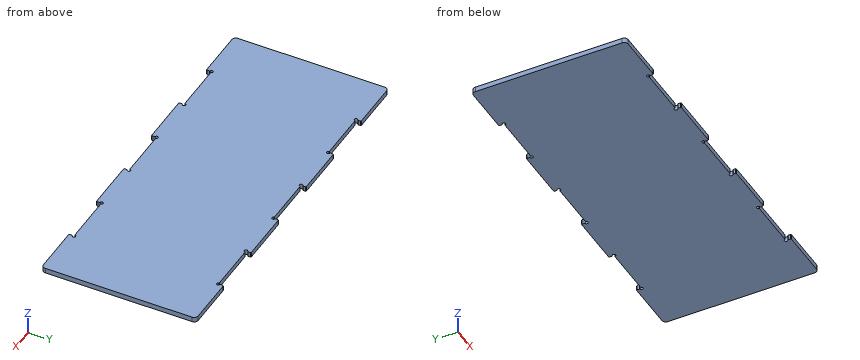
```python
from build123d import *

# Parameters (mm, degrees)
SKETCH1_W               = 455
SKETCH1_H               = 180
BOSS_EXTRUDE1_DEPTH     = 3.175
SKETCH2_W               = 65
SKETCH2_H               = 6.35
BOSS_EXTRUDE2_DEPTH     = 6.35
LPATTERN1_COUNT         = 4
LPATTERN1_PITCH         = 130
MIRROR1_COPY_1_SKETCH_W = 65
MIRROR1_COPY_1_SKETCH_H = 6.35
MIRROR1_COPY_1_DEPTH    = 6.35
MIRROR1_COPY_2_SKETCH_W = 65
MIRROR1_COPY_2_SKETCH_H = 6.35
MIRROR1_COPY_2_DEPTH    = 6.35
MIRROR1_COPY_3_SKETCH_W = 65
MIRROR1_COPY_3_SKETCH_H = 6.35
MIRROR1_COPY_3_DEPTH    = 6.35
SKETCH3_R               = 2
CUT_EXTRUDE1_DEPTH      = 7.35
FILLET2_R               = 1
CUT_EXTRUDE2_DEPTH      = 7.35
LPATTERN2_COUNT         = 3
LPATTERN2_PITCH         = 130
MIRROR2_COPY_1_DEPTH    = 7.35
MIRROR2_COPY_2_DEPTH    = 7.35
FILLET4_R               = 5


with BuildPart() as part:
    # Sketch1 → Boss-Extrude1 (new body, symmetric)
    with BuildSketch(Plane.XY):
        with Locations((227.5, 90)):
            Rectangle(SKETCH1_W, SKETCH1_H)
    extrude(amount=BOSS_EXTRUDE1_DEPTH, both=True)

    # Sketch2 → Boss-Extrude2 (add)
    with BuildSketch(Plane.XY.offset(3.175)):
        with Locations((422.5, -3.175)):
            Rectangle(SKETCH2_W, SKETCH2_H)
    boss_extrude2 = extrude(amount=-BOSS_EXTRUDE2_DEPTH)

    # LPattern1: Boss-Extrude2 ×4
    with Locations(*[(-i * LPATTERN1_PITCH, 0, 0) for i in range(1, LPATTERN1_COUNT)]):
        add(boss_extrude2)

    # Mirror1: Boss-Extrude2 across plane
    add(boss_extrude2.mirror(Plane(origin=(0, 90, 0), x_dir=(0, 0, 1), z_dir=(0, -1, 0))))

    # Mirror1 copy 1 sketch → Mirror1 copy 1 (add)
    with BuildSketch(Plane(origin=(-130, 180, 3.175), x_dir=(1, 0, 0), z_dir=(0, 0, 1))):
        with Locations((422.5, 3.175)):
            Rectangle(MIRROR1_COPY_1_SKETCH_W, MIRROR1_COPY_1_SKETCH_H)
    extrude(amount=-MIRROR1_COPY_1_DEPTH)

    # Mirror1 copy 2 sketch → Mirror1 copy 2 (add)
    with BuildSketch(Plane(origin=(-260, 180, 3.175), x_dir=(1, 0, 0), z_dir=(0, 0, 1))):
        with Locations((422.5, 3.175)):
            Rectangle(MIRROR1_COPY_2_SKETCH_W, MIRROR1_COPY_2_SKETCH_H)
    extrude(amount=-MIRROR1_COPY_2_DEPTH)

    # Mirror1 copy 3 sketch → Mirror1 copy 3 (add)
    with BuildSketch(Plane(origin=(-390, 180, 3.175), x_dir=(1, 0, 0), z_dir=(0, 0, 1))):
        with Locations((422.5, 3.175)):
            Rectangle(MIRROR1_COPY_3_SKETCH_W, MIRROR1_COPY_3_SKETCH_H)
    extrude(amount=-MIRROR1_COPY_3_DEPTH)

    # Sketch3 → Cut-Extrude1 (cut, through all)
    with BuildSketch(Plane.XY.offset(3.175)):
        with Locations((325, 0)):
            Circle(SKETCH3_R)
        with Locations((390, 0)):
            Circle(SKETCH3_R)
    extrude(amount=-CUT_EXTRUDE1_DEPTH, mode=Mode.SUBTRACT)

    # Fillet2
    fillet2_edges = [part.edges().sort_by_distance(p)[0] for p in [
        (390, -6.35, 0),
        (325, -6.35, 0),
    ]]
    fillet(fillet2_edges, radius=FILLET2_R)

    # Sketch4 → Cut-Extrude2 (cut, through all)
    with BuildSketch(Plane.XY.offset(3.175)):
        with BuildLine():
            Line((390, -2.828427125), (390, -5.35))
            ThreePointArc((390, -5.35), (390.292893219, -6.057106781), (391, -6.35))
            Line((391, -6.35), (324, -6.35))
            ThreePointArc((324, -6.35), (324.707106781, -6.057106781), (325, -5.35))
            Line((325, -5.35), (325, -2.828427125))
            ThreePointArc((325, -2.828427125), (324.816496581, -2.251076856), (324.333333333, -1.885618083))
            ThreePointArc((324.333333333, -1.885618083), (323.585786438, 1.414213562), (326.885618083, 0.666666667))
            ThreePointArc((326.885618083, 0.666666667), (327.251076856, 0.183503419), (327.828427125, 0))
            Line((327.828427125, 0), (387.171572875, 0))
            ThreePointArc((387.171572875, 0), (387.748923144, 0.183503419), (388.114381917, 0.666666667))
            ThreePointArc((388.114381917, 0.666666667), (391.414213562, 1.414213562), (390.666666667, -1.885618083))
            ThreePointArc((390.666666667, -1.885618083), (390.183503419, -2.251076856), (390, -2.828427125))
        make_face()
    cut_extrude2 = extrude(amount=-CUT_EXTRUDE2_DEPTH, mode=Mode.SUBTRACT)

    # LPattern2: Cut-Extrude2 ×3
    with Locations(*[(-i * LPATTERN2_PITCH, 0, 0) for i in range(1, LPATTERN2_COUNT)]):
        add(cut_extrude2, mode=Mode.SUBTRACT)

    # Mirror2: Cut-Extrude2 across plane
    add(cut_extrude2.mirror(Plane(origin=(0, 90, 0), x_dir=(0, 0, 1), z_dir=(0, -1, 0))), mode=Mode.SUBTRACT)

    # Mirror2 copy 1 sketch → Mirror2 copy 1 (cut, through all)
    with BuildSketch(Plane(origin=(-130, 180, 3.175), x_dir=(1, 0, 0), z_dir=(0, 0, 1))):
        with BuildLine():
            Line((390, 2.828427125), (390, 5.35))
            ThreePointArc((390, 5.35), (390.292893219, 6.057106781), (391, 6.35))
            Line((391, 6.35), (324, 6.35))
            ThreePointArc((324, 6.35), (324.707106781, 6.057106781), (325, 5.35))
            Line((325, 5.35), (325, 2.828427125))
            ThreePointArc((325, 2.828427125), (324.816496581, 2.251076856), (324.333333333, 1.885618083))
            ThreePointArc((324.333333333, 1.885618083), (323.585786438, -1.414213562), (326.885618083, -0.666666667))
            ThreePointArc((326.885618083, -0.666666667), (327.251076856, -0.183503419), (327.828427125, 0))
            Line((327.828427125, 0), (387.171572875, 0))
            ThreePointArc((387.171572875, 0), (387.748923144, -0.183503419), (388.114381917, -0.666666667))
            ThreePointArc((388.114381917, -0.666666667), (391.414213562, -1.414213562), (390.666666667, 1.885618083))
            ThreePointArc((390.666666667, 1.885618083), (390.183503419, 2.251076856), (390, 2.828427125))
        make_face()
    extrude(amount=-MIRROR2_COPY_1_DEPTH, mode=Mode.SUBTRACT)

    # Mirror2 copy 2 sketch → Mirror2 copy 2 (cut, through all)
    with BuildSketch(Plane(origin=(-260, 180, 3.175), x_dir=(1, 0, 0), z_dir=(0, 0, 1))):
        with BuildLine():
            Line((390, 2.828427125), (390, 5.35))
            ThreePointArc((390, 5.35), (390.292893219, 6.057106781), (391, 6.35))
            Line((391, 6.35), (324, 6.35))
            ThreePointArc((324, 6.35), (324.707106781, 6.057106781), (325, 5.35))
            Line((325, 5.35), (325, 2.828427125))
            ThreePointArc((325, 2.828427125), (324.816496581, 2.251076856), (324.333333333, 1.885618083))
            ThreePointArc((324.333333333, 1.885618083), (323.585786438, -1.414213562), (326.885618083, -0.666666667))
            ThreePointArc((326.885618083, -0.666666667), (327.251076856, -0.183503419), (327.828427125, 0))
            Line((327.828427125, 0), (387.171572875, 0))
            ThreePointArc((387.171572875, 0), (387.748923144, -0.183503419), (388.114381917, -0.666666667))
            ThreePointArc((388.114381917, -0.666666667), (391.414213562, -1.414213562), (390.666666667, 1.885618083))
            ThreePointArc((390.666666667, 1.885618083), (390.183503419, 2.251076856), (390, 2.828427125))
        make_face()
    extrude(amount=-MIRROR2_COPY_2_DEPTH, mode=Mode.SUBTRACT)

    # Fillet4
    fillet4_edges = [part.edges().sort_by_distance(p)[0] for p in [
        (455, -6.35, 0),
        (0, -6.35, 0),
        (455, 186.35, 0),
        (0, 186.35, 0),
    ]]
    fillet(fillet4_edges, radius=FILLET4_R)


solid = part.part
```
Build history of the part. All positions in model axes, mm. Round coordinates to 2 decimals unless told otherwise and drop trailing zeros. Write each loop counter-clockwise with the first axis right and the second up, starting at its lowest first coordinate (ties: lowest second). Pieces come first, ordered by that corner, then holes.
1) Drill centre line: probe 1 along Y at (x, z) = (90, -1.75). Where is it in solid material? Low to high.
2) Pin check, flat tips, straight feed: pin 1 (0.8 mm diameter, centred on y = 184.5, z = 0.5, fed in from -X); pin 2 (3.5 mm diameter, centred on x = 195, y = 0, fed in from -Z); pin 3 (1.3 mm diameter, centred on y = 184, z = 0.5, fed in from -X); pin 4 (0.8 mm diameter, centred on y = 183.5, z = -0.5, fed in from +X). Stop position of each tip, or through.
3) Band-saw the part on A-A, the plane x = 73. List the corners of the cut face in (y, z) (3 decimals).
Ans:
1. probe 1: y = 0 to 180
2. pin 1: stops at x = 0.82
2. pin 2: passes through
2. pin 3: stops at x = 0.42
2. pin 4: stops at x = 454.68
3. outline: (0, -3.175) - (180, -3.175) - (180, 3.175) - (0, 3.175) - close
